For this review, use the dimensioned drawing (mm, ordinates from the lowest corner) and the shaded views. Round coordinates to 2 decimals unless told otherwise and drop trailing zeros. Loops run counter-clockwise (first coordinate to the right, second up) from the corner with the lowest first, then second, coordinate; pieces in that order, holes last. Notation, with made-up numbers: (85.25, 68) - (120.25, 68) arc R11 ccw to (120.25, 80) - close; hole circle Ø5 at (21.25, -8.5). An arc over 180 degrees is marked (long way). Use one line per item in the form item = value. Start each with the question number.
(1) For pin 1 (4 mm diameter, centred on x = 11, y = 5, fed in from -Z); pin 2 (4 mm diameter, centred on y = 12, z = 6.5, fed in from -X); pin 3 (9.5 mm diameter, centred on x = 249.5, y = 5.5, fed in from -Z), all flat-tipped, find the tip position at first contact; note any pin that passes through.
(2) We need section C-C, the plane y = 5.5. Give the number of separate pieces and of enclosed holes in the cut face, then the cut area to 3 significant figures.
(3) We need section B-B, the plane x = 34. Write out the cut boundary in (y, z).
(4) Wall thickness on probe 1 along X at (y, z) = (3.5, 43.5); probe 2 along Z at (x, y) = (241, 1.5); probe 3 along X at (y, z) = (5.75, 386): over which ranges is each line inside the solid? List them lowest first. Write a range as [from, to].
(5) We need section A-A, the plane z = 367. Write out the cut boundary in (x, y), then the cut area to 3 significant figures.
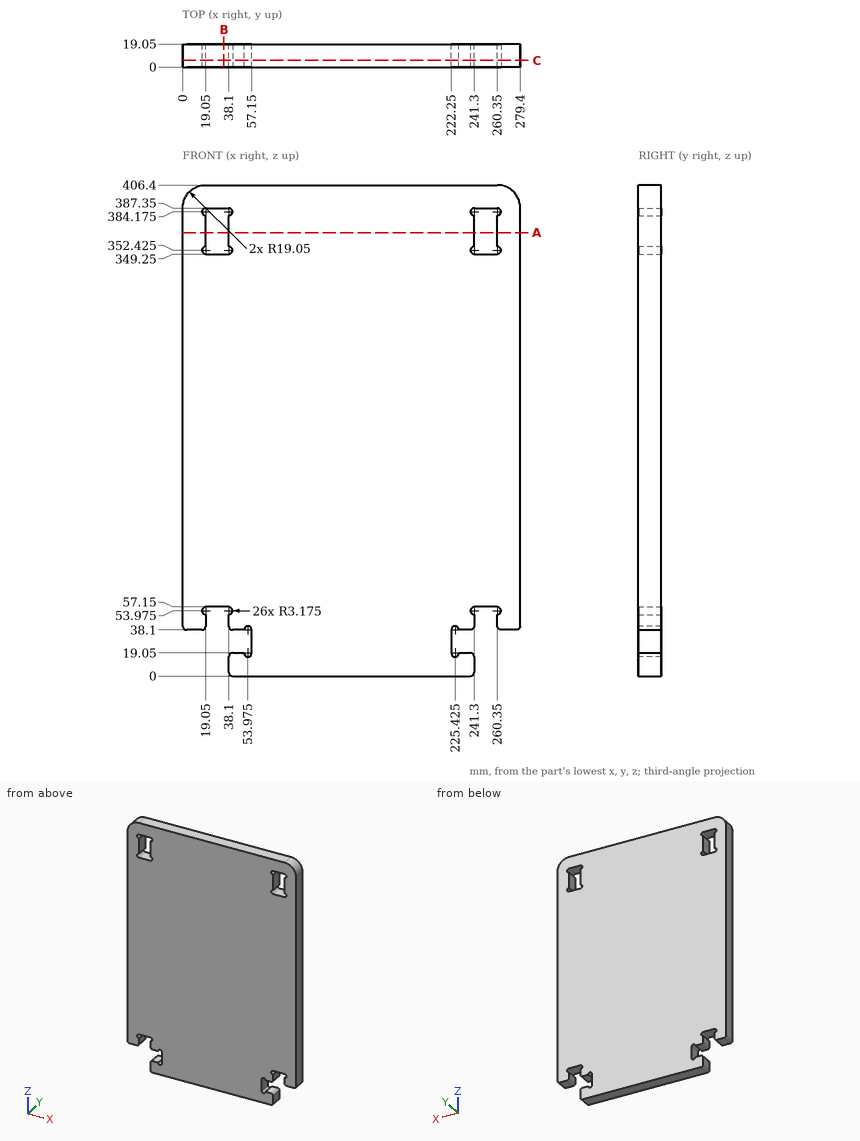
Data:
q1.pin_1 = 38.1
q1.pin_2 = 38.1
q1.pin_3 = 57.15
q2.separate_pieces = 1
q2.enclosed_holes = 2
q2.area = 107,000 mm^2
q3.outline = (0, 57.15) - (19.05, 57.15) - (19.05, 349.25) - (0, 349.25) - close; (0, 387.35) - (19.05, 387.35) - (19.05, 406.4) - (0, 406.4) - close
q4.probe_1 = [0, 19.05], [38.1, 241.3], [260.35, 279.4]
q4.probe_2 = [1.83, 17.22], [39.93, 50.81], [57.14, 349.26], [355.59, 381.01], [387.34, 406.4]
q4.probe_3 = [0, 16.45], [40.7, 238.7], [262.95, 279.4]
q5.outline = (0, 0) - (19.05, 0) - (19.05, 19.05) - (0, 19.05) - close; (38.1, 0) - (241.3, 0) - (241.3, 19.05) - (38.1, 19.05) - close; (260.35, 0) - (279.4, 0) - (279.4, 19.05) - (260.35, 19.05) - close
q5.area = 4,600 mm^2
